from build123d import *

# Parameters (mm, degrees)
SKETCH2_R           = 5
CUT_EXTRUDE1_DEPTH  = 25
SKETCH3_R           = 8
BOSS_EXTRUDE1_DEPTH = 8
SKETCH4_W           = 40
SKETCH4_H           = 12
CUT_EXTRUDE2_DEPTH  = 20


with BuildPart() as part:
    # Sketch1 → Revolve1 (revolve)
    with BuildSketch(Plane(origin=(0, 0, 0), x_dir=(1, 0, 0), z_dir=(0, 1, 0)), mode=Mode.PRIVATE) as revolve1_sk:
        with BuildLine():
            Line((0, 0), (0, 20))
            Line((0, 20), (65, 15))
            ThreePointArc((65, 15), (75.606601718, 10.606601718), (80, 0))
            Line((80, 0), (0, 0))
        make_face()
    revolve(revolve1_sk.sketch.rotate(Axis((-20.908281483, 0, 0), (1, 0, 0)), 180), axis=Axis((-20.908281483, 0, 0), (1, 0, 0)))

    # Sketch2 → Cut-Extrude1 (cut, symmetric)
    with BuildSketch(Plane(origin=(0, 0, 0), x_dir=(1, 0, 0), z_dir=(0, 1, 0))):
        with Locations(Location((65, 0, 0), (0, 0, 270))):
            Circle(SKETCH2_R)
    extrude(amount=CUT_EXTRUDE1_DEPTH, both=True, mode=Mode.SUBTRACT)

    # Sketch3 → Boss-Extrude1 (add)
    with BuildSketch(Plane.ZY):
        with Locations(Location((0, 0, 0), (0, 0, 180))):
            Circle(SKETCH3_R)
    extrude(amount=BOSS_EXTRUDE1_DEPTH)

    # Sketch4 → Cut-Extrude2 (cut, symmetric)
    with BuildSketch(Plane.XY):
        with Locations((65, 0)):
            Rectangle(SKETCH4_W, SKETCH4_H)
    extrude(amount=CUT_EXTRUDE2_DEPTH, both=True, mode=Mode.SUBTRACT)


solid = part.part
Could you check a few things on this model? Use its own coordinates, in mm. A direction names the side the tool comes from. Give positions to 0.01 mm unless a question says otherwise; leave off trailing zeros. Order: outer loops, then holes, each group sorted by start corner. A loop starts at its lowest first (then second) coordinate and runs counter-clockwise, first axis right, second up. Notation, with made-up numbers: (68, 64.5) -> (79, 64.5) arc R19 cw to (79, 75.5) -> close; hole circle Ø1 at (53, -31.75). An arc over 180 degrees is marked (long way). Answer in a Markdown table with one row per item. Add a question column.
Item 1: I'm going to push flat-ended pins straight in: P1, Ø3, axis at x = 69.5, y = -3, coming from the +Z side; P2, Ø8, axis at y = -10, z = 13, coming from the -X side; P3, Ø15.5, axis at x = 54, z = -6.5, coming from the -Y side; P4, Ø3, axis at x = 49, z = 0.5, coming from the -Y side. Where does each tip first touch, or does it pass through?
Item 2: Please list where these lines run through material, in increasing order: probe 1 along X at (y, z) = (-2, 16); probe 2 along X at (y, z) = (3, 0.5); probe 3 along X at (y, z) = (-11, 0).
Item 3: For faces 4 (the flat face through (0, 0, -9)), 5 (the flat face through (45, 0, 0)), 6 (the cylindrical face through (60.12, 10.76, -1.08)), which set-ups out of +Z, -Z, +X, -X, +Y, -Y let a thin tool reach every point of the face, with its end or its side?
Item 4: We'd pull the mould along Y, two halves only. Please class faces 1 (the conical face through (32.96, 17.05, -3.79)), 2 (the cylindrical face through (60.12, -10.63, -1.08)), 3 (the flat face through (58, 6, 0)): pulls with the +Y half, pulls with the -Y half, needs draft (parallel to the pull), parting line crosses it, or undercut.
Item 5: Imagine slicing it at D-D (x = 35.5). List the corners of the cut face in (y, z) for me.
Item 6: Imagine slicing it at B-B (y = 0). List the corners of the cut face in (x, z) for me.
Item 7: Imagine slicing it at A-A (z = 0). List the corners of the cut face in (x, y) for me, and give its area (3 significant figures).
Item 8: Imagine slicing it at C-C (x = 10.5). List the corners of the cut face in (y, z) for me.
Result:
| question | item | result |
|---|---|---|
| 1 | P1 | through |
| 1 | P2 | x = 0 |
| 1 | P3 | y = -16.24 |
| 1 | P4 | y = -16.34 |
| 2 | probe 1 | 0 to 45 |
| 2 | probe 2 | -8 to 45 |
| 2 | probe 3 | 0 to 60, 70 to 75.2 |
| 3 | face 4 | -X |
| 3 | face 5 | +Z, -Z, +X |
| 3 | face 6 | +Y, -Y |
| 4 | face 1 | parting line crosses it |
| 4 | face 2 | needs draft |
| 4 | face 3 | undercut |
| 5 | outline | circle Ø34.54 at (0, 0) |
| 6 | outline | (-8, -8) -> (0, -8) -> (0, -20) -> (45, -16.54) -> (45, 16.54) -> (0, 20) -> (0, 8) -> (-8, 8) -> close |
| 7 | outline | (-8, -8) -> (0, -8) -> (0, -20) -> (60, -15.38) -> (60, -6) -> (45, -6) -> (45, 6) -> (60, 6) -> (60, 15.38) -> (0, 20) -> (0, 8) -> (-8, 8) -> close; (70, -14.14) arc R15 ccw to (78.75, -6) -> (70, -6) -> close; (70, 6) -> (78.75, 6) arc R15 ccw to (70, 14.14) -> close |
| 7 | area | 2,160 mm2 |
| 8 | outline | circle Ø38.38 at (0, 0) |
